Part print with two shaded views. Sizes in mm from the minimum x, y, z corner. A direction names the side the tool comes from. Coordinates: 2 decimals unless noted, no trailing zeros. Order: outer loops, then holes, each group sorted by start corner. A loop starts at its lowest first (then second) coordinate and runs counter-clockwise, first axis right, second up. Notation, with made-up numbers: (-5.75, -28.75) - (48.25, -28.75) arc R16 ccw to (48.25, -19.75) - close; hole circle Ø11 at (17.25, 63.5). An arc over 180 degrees is marked (long way). Write each question's results on one line, items separated by ' | '. Start each with the question number.
Q1. Band-saw the part on A-A, the plane z = 14. Write the cut outline in (x, y).
Q2. Pull direction Y, two halves, no side cores. Call the marked faces 3, 4, 5 and 6: released by +Y, released by -Y, zero draft, split by the parting line, or undercut.
Q3. Band-saw the part on C-C, the plane y = 3.5. Write the cut outline in (x, z).
Q4. Pin check, flat tips, straight feed: P1, Ø3, axis at x = 14, y = 9.5, coming from the -Z side; P2, Ø5.5, axis at x = 14, y = 9.5, coming from the -Z side; P3, Ø5, axis at x = 8.3, z = 23.87, coming from the +Y side; P4, Ø2, axis at x = 19.5, y = 4, coming from the +Z side. Stop position of each tip, or through.
Q5. Which spindle directions (+Z, -Z, +X, -X, +Y, -Y) get a long thin tool onto all of the face, cutting with end or side? Do the marked faces 1 and 2. Say none if no direction does.
Q6. Band-saw the part on B-B, the plane y = 10.5. Write the cut outline in (x, z) (1 decimal), then the cut area to 3 significant figures.
Q7. Band-saw the part on D-D, the plane x = 16.5. Write the cut outline in (y, z) (1 decimal), then the cut area to 3 significant figures.
Q8. Wall check: probe 1 along X at (y, z) = (2.15, 14); probe 2 along Y at (x, z) = (14, 17.5). Give the ranges that are in metal, low to high.
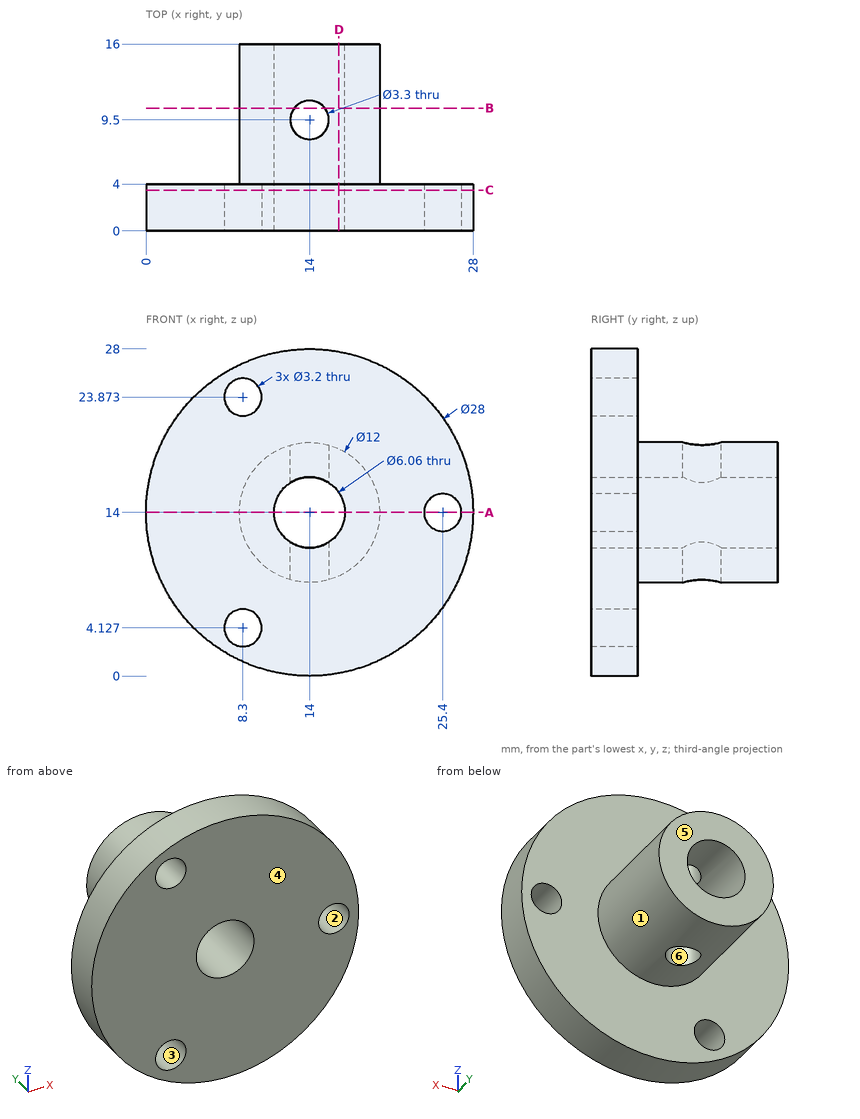
Results below:
1) outline: (0, 0) - (10.97, 0) - (10.97, 16) - (8, 16) - (8, 4) - (0, 4) - close; (17.03, 0) - (23.8, 0) - (23.8, 4) - (20, 4) - (20, 16) - (17.03, 16) - close; (27, 0) - (28, 0) - (28, 4) - (27, 4) - close
2) face 3: zero draft | face 4: released by -Y | face 5: released by +Y | face 6: undercut
3) outline: circle Ø28 at (14, 14); hole circle Ø3.2 at (8.3, 4.13); hole circle Ø3.2 at (8.3, 23.87); hole circle Ø6.06 at (14, 14); hole circle Ø3.2 at (25.4, 14)
4) P1: passes through | P2: stops at z = 8 | P3: stops at y = 4 | P4: stops at z = 27.26
5) face 1: +Y | face 2: +Y, -Y
6) outline: (12.7, 8.1) - (12.7, 11.3) arc R3 cw to (12.7, 16.7) - (12.7, 19.9) arc R6 ccw to start; (15.3, 8.1) arc R6 ccw to (15.3, 19.9) - (15.3, 16.7) arc R3 cw to (15.3, 11.3) - close | area: 68.4 mm²
7) outline: (0, 0.2) - (4, 0.2) - (4, 8.5) - (16, 8.5) - (16, 12.3) - (0, 12.3) - close; (0, 15.7) - (16, 15.7) - (16, 19.5) - (4, 19.5) - (4, 27.8) - (0, 27.8) - close | area: 186 mm²
8) probe 1: x = 0 to 10.97, 17.03 to 23.8, 27 to 28 | probe 2: y = 0 to 7.85, 11.15 to 16
